Geometry: final body of the model. Coordinates: model frame, mm. Coordinates: 2 decimals unless noted, no trailing zeros. Write each loop counter-clockwise with the first axis right and the second up, starting at its lowest first coordinate (ties: lowest second). Pieces come first, ordered by that corner, then holes. Notation, with made-up numbers: M -23,53 L 28,53 A20 ccw 28,85 Z; hole C 55,5 d9. An arc over 180 degrees is marked long. Write item = value, one per line. Start each with the question number.
Item 1: Section B-B on x = 0. Output: boundary loops of the cut face in (y, z).
Item 2: Pull-direction query (Z, two-part tool) for faces 1 (the cylindrical face through (-1.893, -1.916, 13.164)), 2 (the cylindrical face through (28.55, -0.09, 11.94)), 3 (the flat face through (-8, 6.35, 5)), 4 (the flat face through (0, 0, 19.05)); classes: +Z half, -Z half, draft (parallel to the pull), parting line (faces both ways), or undercut.
Item 3: Ray query, L1, parallel to X at y = 5, z = 12.5 (3 decimals); L2, parallel to Z at x = 0, y = 0; L3, parallel to X at y = 0, z = 7 (3 decimals). Return the intervals inside material, ascending. Write a range as [from, to].
Item 4: Section A-A on x = -25.4. Output: boundary loops of the cut face in (y, z), plus the area to 3 significant figures.
Item 5: Section C-C on y = 2. Give the number of separate pieces and of enclosed holes in the cut face, plus the area to 3 significant figures.
from build123d import *

# Parameters (mm, degrees)
SKETCH1_W                                           = 69.85
SKETCH1_H                                           = 12.7
BOSS_EXTRUDE1_DEPTH                                 = 19.05
F_5_16_0_3125_DIAMETER_HOLE1_D                      = 7.9375
CSK_FOR_5_16_FLAT_HEAD_MACHINE_SCREW_10_D           = 8.2042
CSK_FOR_5_16_FLAT_HEAD_MACHINE_SCREW_10_CSINK_D     = 17.0371262
CSK_FOR_5_16_FLAT_HEAD_MACHINE_SCREW_10_CSINK_ANGLE = 100


with BuildPart() as part:
    # Sketch1 → Boss-Extrude1 (new body)
    with BuildSketch(Plane.XY):
        Rectangle(SKETCH1_W, SKETCH1_H)
    extrude(amount=BOSS_EXTRUDE1_DEPTH)

    # 5/16 (0.3125) Diameter Hole1 (through all)
    with Locations(Plane(origin=(0, 6.35, 0), x_dir=(1, 0, 0), z_dir=(0, 1, 0))):
        with Locations((-25.4, -9.525), (25.4, -9.525)):
            Hole(F_5_16_0_3125_DIAMETER_HOLE1_D / 2)

    # CSK for 5/16 Flat Head Machine Screw (100)1 (through all)
    with Locations(Plane(origin=(0, 6.35, 0), x_dir=(1, 0, 0), z_dir=(0, 1, 0))):
        with Locations((0, -9.525)):
            CounterSinkHole(CSK_FOR_5_16_FLAT_HEAD_MACHINE_SCREW_10_D / 2, CSK_FOR_5_16_FLAT_HEAD_MACHINE_SCREW_10_CSINK_D / 2, counter_sink_angle=CSK_FOR_5_16_FLAT_HEAD_MACHINE_SCREW_10_CSINK_ANGLE)


solid = part.part
Responses:
q1.outline = M -6.35,0 L 6.35,0 L 6.35,1.01 L 2.64,5.42 L -6.35,5.42 Z; M -6.35,13.63 L 2.64,13.63 L 6.35,18.04 L 6.35,19.05 L -6.35,19.05 Z
q2.face_1 = undercut
q2.face_2 = undercut
q2.face_3 = draft
q2.face_4 = +Z half
q3.L1 = [-34.925, -28.027], [-22.773, -6.236], [6.236, 22.773], [28.027, 34.925]
q3.L2 = [0, 5.42], [13.63, 19.05]
q3.L3 = [-34.925, -28.462], [-22.338, -3.233], [3.233, 22.338], [28.462, 34.925]
q4.outline = M -6.35,0 L 6.35,0 L 6.35,5.56 L -6.35,5.56 Z; M -6.35,13.49 L 6.35,13.49 L 6.35,19.05 L -6.35,19.05 Z
q4.area = 141 mm²
q5.separate_pieces = 1
q5.enclosed_holes = 3
q5.area = 1,180 mm²
